Geometry: final body of the model. Coordinates: model frame, mm. A direction names the side the tool comes from. Coordinates: 2 decimals unless noted, no trailing zeros. Loops run counter-clockwise (first coordinate to the right, second up) from the corner with the lowest first, then second, coordinate; pieces in that order, holes last. Notation, with made-up numbers: (21, 47) - (39, 47) arc R30 ccw to (39, 85) - close; hole circle Ø11 at (82.5, 35). An arc over 180 degrees is marked (long way). Return JSON: item names as keys, results as strings.
from build123d import *

# Parameters (mm, degrees)
F1_DEPTH = 1.5875
F3_DEPTH = 6.35
F4_R     = 3.175
F5_DEPTH = 28.575


with BuildPart() as f1:
    # F0 (on Top) → F1 (new body)
    with BuildSketch(Plane.XY):
        Polygon((8.382, -10.31875), (8.382, 15.875), (-8.382, 10.31875), (-8.382, -15.875), align=None)
    extrude(amount=-F1_DEPTH)

    # F2 (on face) → F3 (join)
    with BuildSketch(Plane.XY):
        with BuildLine():
            Line((6.600987, -10.909048), (-3.519459, -14.263362))
            ThreePointArc((-3.519459, -14.263362), (2.277457, -14.808913), (6.600987, -10.909048))
        make_face()
        with BuildLine():
            ThreePointArc((6.600987, -10.909048), (7.0777, -9.457135), (7.239, -7.9375))
            ThreePointArc((7.239, -7.9375), (-3.66918, -1.697288), (-3.519459, -14.263362))
            Line((-3.519459, -14.263362), (6.600987, -10.909048))
        make_face()
    extrude(amount=F3_DEPTH)

    # F4 (on Top) → F5 (join)
    with BuildSketch(Plane.XY):
        with Locations((0, -7.9375)):
            Circle(F4_R)
    extrude(amount=F5_DEPTH)


solid = f1.part
Item 1: Section query A-A, the plane x = -5.75. Return loops of the section in (y, z), and give its area (3 significant figures).
Worked out:
{"outline": "(-15, -1.59) - (11.19, -1.59) - (11.19, 0) - (-3.54, 0) - (-3.54, 6.35) - (-12.34, 6.35) - (-12.34, 0) - (-15, 0) - close", "area": "97.4 mm^2"}
Item 2: Ray query, probe 1 along Z at (x, y) = (-5.25, 1.5); probe 2 along Z at (x, y) = (-2.75, -10); probe 3 along X at (y, z) = (-10.5, 18). Return the intervals inside material, ascending. Write a range as from..to.
Worked out:
{"probe 1": "-1.59..0", "probe 2": "-1.59..6.35", "probe 3": "-1.87..1.87"}
Item 3: Section query D-D, the plane y = -12.5. Return loops of the section in (x, z).
Worked out:
{"outline": "(-8.38, -1.59) - (1.8, -1.59) - (1.8, 0) - (5.62, 0) - (5.62, 6.35) - (-5.62, 6.35) - (-5.62, 0) - (-8.38, 0) - close"}
Item 4: First-contact query: pin 1 Ø8 at (x, z) = (6, 4.5) entering from +Y; pin 2 Ø5 at (y, z) = (-8.5, 5) entering from +X; pin 3 Ø10 at (x, y) = (-2.5, 7) entering from +Z. Flat tips, straight axial feed; report the tip coordinate or a pass-through.
Worked out:
{"pin 1": "y = -0.98", "pin 2": "x = 7.24", "pin 3": "z = 0"}
Item 5: Reachability of faces 1 (the face through (7.073, -9.478, 3.131)), 2 (the face through (-0.688, -11.037, 17.307)), 3 (the face through (1, -13, 0)) from +Z, -Z, +X, -X, +Y, -Y: full face, straight path, thin tool, end or side. Return the list, or none.
Worked out:
{"face 1": "+Z, +X, -Y", "face 2": "+Z", "face 3": "-Z, +X, -Y"}
